Here's how the part is built. I have some questions about the finished solid (model axes, mm). Face numbers are marked on the shaded views. Round coordinates to 2 decimals unless told otherwise and drop trailing zeros. One line per item, written item: value. Start each with the question number.
```python
from build123d import *

# Parameters (mm, degrees)
SKETCH_1_W                = 176
SKETCH_1_H                = 178
EXTRUDE_1_DEPTH           = 12.6
EXTRUDE_3_DEPTH           = 2.4
SKETCH_8_W                = 5
SKETCH_8_H                = 5
CUT_EXTRUDE_4_DEPTH       = 2.4
HOLE_WIZARD_M4_1_D        = 3.3
HOLE_WIZARD_M4_1_DEPTH    = 5
HOLE_WIZARD_M4_1_TIP      = 0.991420021
SKETCH_14_W               = 5
SKETCH_14_H               = 6.6
CUT_EXTRUDE_6_DEPTH       = 177
SKETCH_15_W               = 3
SKETCH_15_H               = 9.6
CUT_EXTRUDE_7_DEPTH       = 177
PATTERN_LINEAR_3_COUNT    = 23
PATTERN_LINEAR_3_PITCH    = 6.136363636
HOLE_WIZARD_2_D           = 6.6
HOLE_WIZARD_2_CBORE_D     = 11
HOLE_WIZARD_2_CBORE_DEPTH = 6.8
MM_2_D                    = 4
MM_2_DEPTH                = 5
MM_2_TIP                  = 1.201721238
CUT_EXTRUDE_11_DEPTH      = 5


with BuildPart() as part:
    # 草图1 → 凸台-拉伸1 (new body)
    with BuildSketch(Plane(origin=(0, 12.6, 0), x_dir=(1, 0, 0), z_dir=(0, 1, 0))):
        with Locations((-15.748130707, -439.724508868)):
            Rectangle(SKETCH_1_W, SKETCH_1_H)
    extrude(amount=-EXTRUDE_1_DEPTH)

    # 草图7 → 凸台-拉伸3 (add)
    with BuildSketch(Plane(origin=(0, 12.6, 0), x_dir=(1, 0, 0), z_dir=(0, 1, 0))):
        Polygon((69.251869293, -528.724508868), (69.251869293, -353.724508868), (-100.748130707, -353.724508868), (-100.748130707, -528.724508868), (-103.748130707, -528.724508868), (-103.748130707, -350.724508868), (72.251869293, -350.724508868), (72.251869293, -528.724508868), align=None)
    extrude(amount=EXTRUDE_3_DEPTH)

    # 草图8 → 切除-拉伸4 (cut)
    with BuildSketch(Plane(origin=(0, 15, 0), x_dir=(1, 0, 0), z_dir=(0, 1, 0))):
        with Locations((-101.248130707, -353.224508868)):
            Rectangle(SKETCH_8_W, SKETCH_8_H)
        with Locations((69.751869293, -353.224508868)):
            Rectangle(SKETCH_8_W, SKETCH_8_H)
    extrude(amount=-CUT_EXTRUDE_4_DEPTH, mode=Mode.SUBTRACT)

    # M4 螺纹孔1
    with Locations(Plane(origin=(-96.748130707, 12.6, 357.724508868), x_dir=(0, 0, 1), z_dir=(0, 1, 0))):
        with Locations((0, 0), (0, 62), (164, 62), (164, 0), (164, 100), (164, 162), (0, 162), (0, 100)):
            Hole(HOLE_WIZARD_M4_1_D / 2, depth=HOLE_WIZARD_M4_1_DEPTH)
            with Locations((0, 0, -(HOLE_WIZARD_M4_1_DEPTH + HOLE_WIZARD_M4_1_TIP / 2))):  # 118° drill point
                Cone(0, HOLE_WIZARD_M4_1_D / 2, HOLE_WIZARD_M4_1_TIP, mode=Mode.SUBTRACT)

    # 草图14 → 切除-拉伸6 (cut, through all)
    with BuildSketch(Plane.ZY.offset(103.748130707)):
        with Locations((526.224508868, 6.3)):
            Rectangle(SKETCH_14_W, SKETCH_14_H)
        with Locations((353.224508868, 6.3)):
            Rectangle(SKETCH_14_W, SKETCH_14_H)
    extrude(amount=-CUT_EXTRUDE_6_DEPTH, mode=Mode.SUBTRACT)

    # 草图15 → 切除-拉伸7 (cut, through all)
    with BuildSketch(Plane.ZY.offset(103.748130707)):
        with Locations((507.224508868, 4.8)):
            Rectangle(SKETCH_15_W, SKETCH_15_H)
    cut_extrude_7 = extrude(amount=-CUT_EXTRUDE_7_DEPTH, mode=Mode.SUBTRACT)

    # 阵列(线性)3: 切除-拉伸7 ×23
    with Locations(*[(0, 0, -i * PATTERN_LINEAR_3_PITCH) for i in range(1, PATTERN_LINEAR_3_COUNT)]):
        add(cut_extrude_7, mode=Mode.SUBTRACT)

    # 打孔尺寸(%根据)内六角圆柱头螺钉的类型2 (through all)
    with Locations(Plane(origin=(-15.748130707, 12.6, 514.724508868), x_dir=(0, 0, 1), z_dir=(0, 1, 0))):
        with Locations((0, 0), (-150, 0)):
            CounterBoreHole(HOLE_WIZARD_2_D / 2, HOLE_WIZARD_2_CBORE_D / 2, HOLE_WIZARD_2_CBORE_DEPTH)

    # 大小mm 暗销孔2
    with Locations(Plane(origin=(-5.748130707, 0, 364.724508868), x_dir=(0, 0, -1), z_dir=(0, -1, 0))):
        with Locations((0, 0)):
            Hole(MM_2_D / 2, depth=MM_2_DEPTH)
            with Locations((0, 0, -(MM_2_DEPTH + MM_2_TIP / 2))):  # 118° drill point
                Cone(0, MM_2_D / 2, MM_2_TIP, mode=Mode.SUBTRACT)

    # 草图22 → 切除-拉伸11 (cut)
    with BuildSketch(Plane.XZ):
        with BuildLine():
            Line((-7.748130707, 513.724508868), (-7.748130707, 515.724508868))
            ThreePointArc((-7.748130707, 515.724508868), (-5.748130707, 517.724508868), (-3.748130707, 515.724508868))
            Line((-3.748130707, 515.724508868), (-3.748130707, 513.724508868))
            ThreePointArc((-3.748130707, 513.724508868), (-5.748130707, 511.724508868), (-7.748130707, 513.724508868))
        make_face()
    extrude(amount=-CUT_EXTRUDE_11_DEPTH, mode=Mode.SUBTRACT)


solid = part.part
```
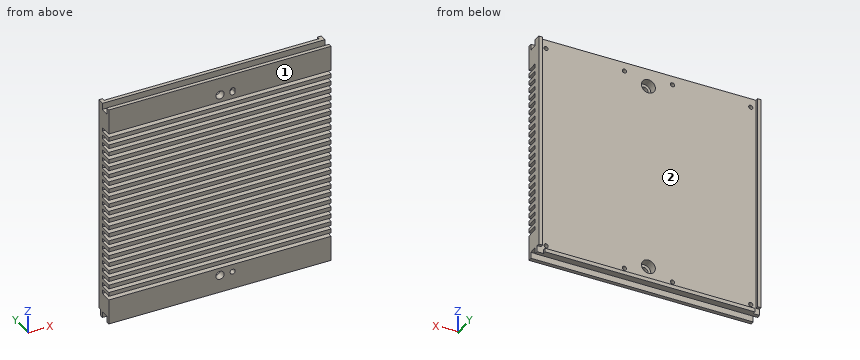
Q1. If I drill on line 1 along X through (y, z) = (4.75, 513.5); line 2 along X through (y, z) = (13.75, 454); line 3 along Z through (x, y) = (64.5, 14), over which ranges is the centre line in solid material (lowest first)?
Q2. If we mould it in two halves opening along X, with no side actions, what happens to the marked faces 1 and 2? For each: released by +X, released by -X, zero draft, split by the parting line, or undercut.
Q3. Will these pins go through, and if not, where does the flat tip stop? P1, Ø4, axis at x = 32, y = 8.5, coming from the +Z side; P2, Ø1.2, axis at x = 24.5, y = 14, coming from the +Z side; P3, Ø3, axis at x = 14, y = 5, coming from the +Z side; P4, Ø1, axis at x = -31.5, z = 485, coming from the +Y side.
Answers below:
1. line 1: x = -103.75 to -18.81, -12.68 to -7.74, -3.76 to 72.25
1. line 2: x = -103.75 to -100.75, 69.25 to 72.25
1. line 3: z = 350.72 to 353.72
2. face 1: zero draft
2. face 2: undercut
3. P1: stops at z = 528.72
3. P2: stops at z = 353.72
3. P3: stops at z = 523.72
3. P4: stops at y = 12.6
